Can you work these out from the model? Positions are in its coordinate system, mm. A direction names the side the tool comes from. Round coordinates to 2 decimals unless told otherwise and drop trailing zeros. Order: outer loops, then holes, each group sorted by start corner. A loop starts at its lowest first (then second) coordinate and runs counter-clockwise, first axis right, second up.
Q1. If we section it at C-C (y = 14): Please give me the cut outline in (x, z), plus the area to 3 significant figures.
Q2. If we section it at B-B (x = 31): Please give me the cut outline in (y, z).
Q3. If we section it at A-A (y = 45): Please give me the cut outline in (x, z), plus the area to 3 significant figures.
Q4. If we section it at D-D (z = 22): Please give me the cut outline in (x, y), plus the area to 3 significant figures.
Q5. For faces 4 (the face through (-43, -6, 5)), 5 (the face through (-2, 41, 5)), 6 (the face through (22.528, 46, 2)), 7 (the face through (42, -33.852, 7)), which set-ups out of +Z, -Z, +X, -X, +Y, -Y let a thin tool reach every point of the face, with its end or its side?
Q6. If I drill on line 1 (Y direction, x = 62, z = 47); line 2 (Z direction, x = -33, y = 3.5); line 3 (Z direction, x = -10.5, y = -54), over which ranges is the centre line in solid material (lowest first)?
Q7. We'd pull the mould along X, two halves only. Please class faces 1 (the face through (-2, -13, 0)), 2 (the face through (-20.712, 46, 2)), 3 (the face through (-70.592, -32, 3)): pulls with the +X half, pulls with the -X half, needs draft (parallel to the pull), parting line crosses it, or undercut.
Q8. Will these pins go through, and if not, where does the flat tip stop? P1, Ø15, axis at x = -2.5, y = -6.5, coming from the +Z side; P2, Ø0.9, axis at x = -22.5, z = 3.5, coming from the +Y side; P3, Ø1.5, axis at x = 33, y = 40.5, coming from the +Z side.
from build123d import *

# Parameters (mm, degrees)
F0_W     = 40.2394990027
F0_H     = 20
F0_W_2   = 55
F0_H_2   = 55
F1_DEPTH = 5
F0_W_3   = 30
F2_DEPTH = 10
F4_DEPTH = 141
F5_DEPTH = 60


# Not quite as in the source:
# - a feature names something its author has since deleted; it is built from what else it names


with BuildPart() as f1:
    # F0 (on Top) → F1 (new body)
    with BuildSketch(Plane.XY):
        with BuildLine():
            Line((-40.5921050906, 26.1479860185), (-65.5921050906, 26.1479860185))
            ThreePointArc((-65.5921050906, 26.1479860185), (-67.0565711847, 22.6124521126), (-70.5921050906, 21.1479860185))
            Line((-70.5921050906, 21.1479860185), (-15.5921050906, 21.1479860185))
            Line((-15.5921050906, 21.1479860185), (14.4078949094, 21.1479860185))
            Line((14.4078949094, 21.1479860185), (69.4078949094, 21.1479860185))
            ThreePointArc((69.4078949094, 21.1479860185), (65.8723610034, 22.6124521126), (64.4078949094, 26.1479860185))
            Line((64.4078949094, 26.1479860185), (39.4078949094, 26.1479860185))
            Line((39.4078949094, 26.1479860185), (-40.5921050906, 26.1479860185))
        make_face()
        with BuildLine():
            Line((-45.5921050906, 56.1479860185), (-70.5921050906, 56.1479860185))
            Line((-70.5921050906, 56.1479860185), (-70.5921050906, 31.1479860185))
            ThreePointArc((-70.5921050906, 31.1479860185), (-67.0565711847, 29.6835199245), (-65.5921050906, 26.1479860185))
            Line((-65.5921050906, 26.1479860185), (-40.5921050906, 26.1479860185))
            Line((-40.5921050906, 26.1479860185), (-40.5921050906, 51.1479860185))
            ThreePointArc((-40.5921050906, 51.1479860185), (-44.1276389966, 52.6124521126), (-45.5921050906, 56.1479860185))
        make_face()
        with Locations((-0.5921050906, 46.1479860185)):
            Rectangle(F0_W, F0_H)
        with BuildLine():
            Line((39.4078949094, 51.1479860185), (39.4078949094, 26.1479860185))
            Line((39.4078949094, 26.1479860185), (64.4078949094, 26.1479860185))
            ThreePointArc((64.4078949094, 26.1479860185), (65.8723610034, 29.6835199245), (69.4078949094, 31.1479860185))
            Line((69.4078949094, 31.1479860185), (69.4078949094, 56.1479860185))
            Line((69.4078949094, 56.1479860185), (44.4078949094, 56.1479860185))
            ThreePointArc((44.4078949094, 56.1479860185), (42.9434288153, 52.6124521126), (39.4078949094, 51.1479860185))
        make_face()
        with BuildLine():
            ThreePointArc((-35.5921050906, 56.1479860185), (-37.0565711847, 52.6124521126), (-40.5921050906, 51.1479860185))
            Line((-40.5921050906, 51.1479860185), (-40.5921050906, 26.1479860185))
            Line((-40.5921050906, 26.1479860185), (39.4078949094, 26.1479860185))
            Line((39.4078949094, 26.1479860185), (39.4078949094, 51.1479860185))
            ThreePointArc((39.4078949094, 51.1479860185), (35.8723610034, 52.6124521126), (34.4078949094, 56.1479860185))
            Line((34.4078949094, 56.1479860185), (22.5276444107, 56.1479860185))
            Line((22.5276444107, 56.1479860185), (22.5276444107, 36.1479860185))
            Line((22.5276444107, 36.1479860185), (19.5276444107, 36.1479860185))
            Line((19.5276444107, 36.1479860185), (-20.711854592, 36.1479860185))
            Line((-20.711854592, 36.1479860185), (-23.711854592, 36.1479860185))
            Line((-23.711854592, 36.1479860185), (-23.711854592, 56.1479860185))
            Line((-23.711854592, 56.1479860185), (-35.5921050906, 56.1479860185))
        make_face()
        with Locations((-43.0921050906, -6.3520139815)):
            Rectangle(F0_W_2, F0_H_2)
        with Locations((41.9078949094, -6.3520139815)):
            Rectangle(F0_W_2, F0_H_2)
    extrude(amount=F1_DEPTH)

    # F0 (on Top) → F2 (join)
    with BuildSketch(Plane.XY):
        with Locations((-0.5921050906, -6.3520139815)):
            Rectangle(F0_W_3, F0_H_2)
        Polygon((-15.5921050906, -33.8520139815), (-70.5921050906, -33.8520139815), (-70.5921050906, -83.8520139815), (69.4078949094, -83.8520139815), (69.4078949094, -33.8520139815), (14.4078949094, -33.8520139815), align=None)
    extrude(amount=F2_DEPTH)

    # F3 (on face) → F4 (cut)
    with BuildSketch(Plane(origin=(-70.5921050906, 0, 0), x_dir=(0, -1, 0), z_dir=(-1, 0, 0))):
        Polygon((83.8520139815, 10), (33.8520139815, 10), (83.8520139815, 0), align=None)
    extrude(amount=-F4_DEPTH, mode=Mode.SUBTRACT)

    # F0 (on Top) → F5 (join)
    with BuildSketch(Plane.XY):
        with BuildLine():
            Line((-40.5921050906, 26.1479860185), (-65.5921050906, 26.1479860185))
            ThreePointArc((-65.5921050906, 26.1479860185), (-67.0565711847, 22.6124521126), (-70.5921050906, 21.1479860185))
            Line((-70.5921050906, 21.1479860185), (-15.5921050906, 21.1479860185))
            Line((-15.5921050906, 21.1479860185), (14.4078949094, 21.1479860185))
            Line((14.4078949094, 21.1479860185), (69.4078949094, 21.1479860185))
            ThreePointArc((69.4078949094, 21.1479860185), (65.8723610034, 22.6124521126), (64.4078949094, 26.1479860185))
            Line((64.4078949094, 26.1479860185), (39.4078949094, 26.1479860185))
            Line((39.4078949094, 26.1479860185), (-40.5921050906, 26.1479860185))
        make_face()
    extrude(amount=F5_DEPTH)


solid = f1.part
Solution:
1. outline: (-70.59, 0) - (69.41, 0) - (69.41, 5) - (14.41, 5) - (14.41, 10) - (-15.59, 10) - (-15.59, 5) - (-70.59, 5) - close
1. area: 850 mm2
2. outline: (-83.85, 0) - (56.15, 0) - (56.15, 5) - (26.15, 5) - (26.15, 60) - (21.15, 60) - (21.15, 5) - (-33.85, 5) - (-33.85, 10) - close
3. outline: (-70.59, 0) - (-23.71, 0) - (-23.71, 5) - (-70.59, 5) - close; (-20.71, 0) - (19.53, 0) - (19.53, 5) - (-20.71, 5) - close; (22.53, 0) - (69.41, 0) - (69.41, 5) - (22.53, 5) - close
3. area: 670 mm2
4. outline: (-70.59, 21.15) - (69.41, 21.15) arc R5 cw to (64.41, 26.15) - (-65.59, 26.15) arc R5 cw to start
4. area: 661 mm2
5. face 4: +Z, -X
5. face 5: +Z, +X, -X, +Y
5. face 6: +Z, -Z, +Y
5. face 7: +Z, +X
6. line 1: y = 21.15 to 26.15
6. line 2: z = 0 to 5
6. line 3: z = 0 to 5.97
7. face 1: needs draft
7. face 2: undercut
7. face 3: pulls with the -X half
8. P1: stops at z = 10
8. P2: stops at y = 36.15
8. P3: stops at z = 5
